Source: CAD feature listing. Evaluate the final solid. Frame: model axes, mm. Face numbers are marked on the shaded views. A direction names the side the tool comes from. Coordinates: 2 decimals unless noted, no trailing zeros. Write each loop counter-clockwise with the first axis right and the second up, starting at its lowest first coordinate (ties: lowest second). Pieces come first, ordered by that corner, then holes. Notation, with made-up numbers: M 37.25,45 L 92.25,45 A26 cw 92.25,74 Z; hole C 11.25,74 d5. An arc over 180 degrees is marked long. Answer as CSV lines item,"result". Start each with the question number.
1. Section C-C on x = 766. Return the cut outline in (y, z), plus the area to 3 significant figures.
2. Section B-B on z = -616.5. Return the cut outline in (x, y).
3. Reachability of the marked faces 5 and 6 from +Z, -Z, +X, -X, +Y, -Y: full face, straight path, thin tool, end or side. Return the list, or none.
4. Line query: probe 1 along X at (y, z) = (506.5, -618); probe 2 along Y at (x, z) = (771, -676). Output: solid intervals per line, ascending. Write a range as [from, to].
5. Mould query, pull axis Y, two halves, no side actions, for the marked faces 1, 2, 3 and 4. Classes: pulls with the +Y half, pulls with the -Y half, needs draft (parallel to the pull), parting line crosses it, or undercut.
6. Section A-A on y = 537. Return the cut outline in (x, z).
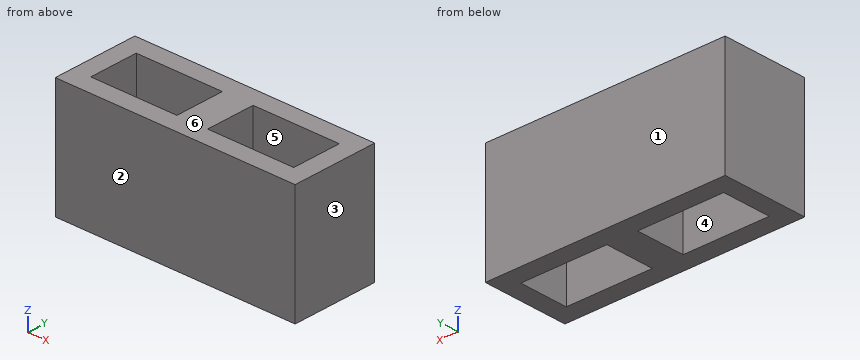
```python
from build123d import *

# Parameters (mm, degrees)
BOX035_W     = 140
BOX035_H     = 80
BOX035_DEPTH = 190
BOX036_W     = 140
BOX036_H     = 80
BOX036_DEPTH = 190
BOX037_W     = 390
BOX037_H     = 140
BOX037_DEPTH = 190


with BuildPart() as cube025:
    # Box035 → Box035 (new body)
    with BuildSketch(Plane(origin=(220, 30, 0), x_dir=(1, 0, 0), z_dir=(0, 0, 1))):
        with Locations((70, 40)):
            Rectangle(BOX035_W, BOX035_H)
    extrude(amount=BOX035_DEPTH)


with BuildPart() as fusion011:
    # Box036 → Box036 (new body)
    with BuildSketch(Plane(origin=(30, 30, 0), x_dir=(1, 0, 0), z_dir=(0, 0, 1))):
        with Locations((70, 40)):
            Rectangle(BOX036_W, BOX036_H)
    extrude(amount=BOX036_DEPTH)

    # Fusion011: union Cube025
    add(cube025.part)


with BuildPart() as cut008:
    # Box037 → Box037 (new body)
    with BuildSketch(Plane.XY):
        with Locations((195, 70)):
            Rectangle(BOX037_W, BOX037_H)
    extrude(amount=BOX037_DEPTH)

    # Cut008: cut Fusion011
    add(fusion011.part, mode=Mode.SUBTRACT)


with BuildPart() as cut008_1:
    # Cut008 placement: moved
    add(cut008.part.moved(Location((630, 445, -790))))


solid = cut008_1.part
```
Values:
1,outline,"M 445,-790 L 475,-790 L 475,-600 L 445,-600 Z; M 555,-790 L 585,-790 L 585,-600 L 555,-600 Z"
1,area,"11,400 mm²"
2,outline,"M 630,445 L 1020,445 L 1020,585 L 630,585 Z; hole M 660,475 L 800,475 L 800,555 L 660,555 Z; hole M 850,475 L 990,475 L 990,555 L 850,555 Z"
3,face 5,"+Z, -Z"
3,face 6,"+Z, +X, -X, +Y, -Y"
4,probe 1,"[630, 660], [800, 850], [990, 1020]"
4,probe 2,"[445, 475], [555, 585]"
5,face 1,"pulls with the +Y half"
5,face 2,"pulls with the -Y half"
5,face 3,"needs draft"
5,face 4,"undercut"
6,outline,"M 630,-790 L 660,-790 L 660,-600 L 630,-600 Z; M 800,-790 L 850,-790 L 850,-600 L 800,-600 Z; M 990,-790 L 1020,-790 L 1020,-600 L 990,-600 Z"
